Source: three-view drawing plus pictorial views. Frame: mm from the lowest corner of the part. A direction names the side the tool comes from. Give positions to 0.01 mm unless a question says otherwise; leave off trailing zeros. Order: outer loops, then holes, each group sorted by start corner. A loop starts at its lowest first (then second) coordinate and runs counter-clockwise, first axis right, second up. Notation, with made-up numbers: (52, 79) - (110, 79) arc R13 ccw to (110, 93) - close; hole circle Ø4 at (44.5, 68). An arc over 180 degrees is marked (long way). Use CSV: the item, a comma, the result in double quotes.
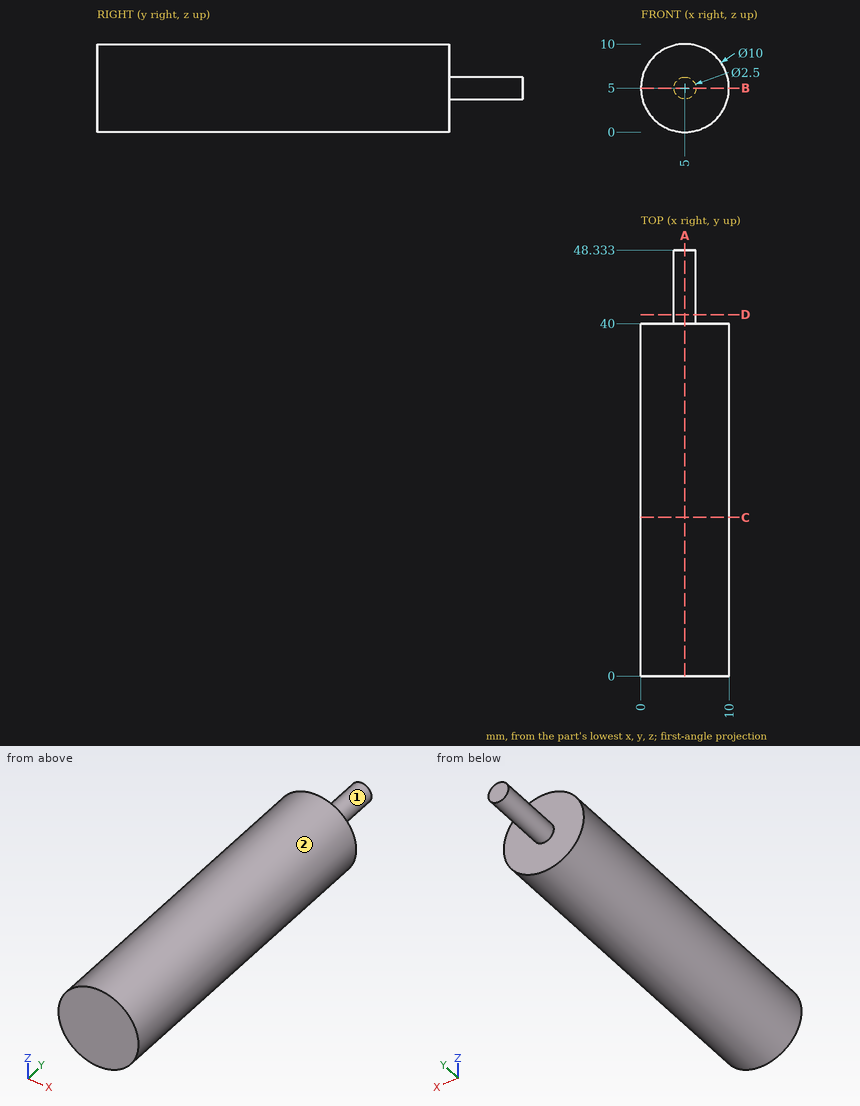
Item 1: Material intervals for line 1 (Y direction, x = 9, z = 7); line 2 (Z direction, x = 4.75, y = 20.5), sorted ascending. Write a range as from..to.
Filled in:
line 1,"y = 0..40"
line 2,"z = 0.01..9.99"
Item 2: Section D-D on y = 41. Return the cut outline in (x, z).
Filled in:
outline,"circle Ø2.5 at (5, 5)"
Item 3: First-contact query: pin 1 (5 mm diameter, centred on x = 2, y = 39, fed in from -Z) (1 decimal); pin 2 (2 mm diameter, centred on y = 10, z = 8.5, fed in from +X); pin 3 (1 mm diameter, centred on y = 22, z = 7, fed in from +X). Flat tips, straight axial feed; report the tip coordinate or a pass-through.
Filled in:
pin 1,"stops at z = 0"
pin 2,"stops at x = 9.33"
pin 3,"stops at x = 9.77"
Item 4: Section A-A on x = 5. Return the cut outline in (y, z).
Filled in:
outline,"(0, 0) - (40, 0) - (40, 3.75) - (48.33, 3.75) - (48.33, 6.25) - (40, 6.25) - (40, 10) - (0, 10) - close"
Item 5: Set-up query: the marked faces 1 and 2. Return all of +Z, -Z, +X, -X, +Y, -Y with unobstructed straight access to the full face (end or side cutting, diameter ignored); none if empty.
Filled in:
face 1,"+Y"
face 2,"+Y, -Y"
Item 6: Section C-C on y = 18. Return the cut outline in (x, z).
Filled in:
outline,"circle Ø10 at (5, 5)"
Item 7: Section B-B on z = 5. Return the cut outline in (x, y), then the cut area to 3 significant figures.
Filled in:
outline,"(0, 0) - (10, 0) - (10, 40) - (6.25, 40) - (6.25, 48.33) - (3.75, 48.33) - (3.75, 40) - (0, 40) - close"
area,"421 mm2"
